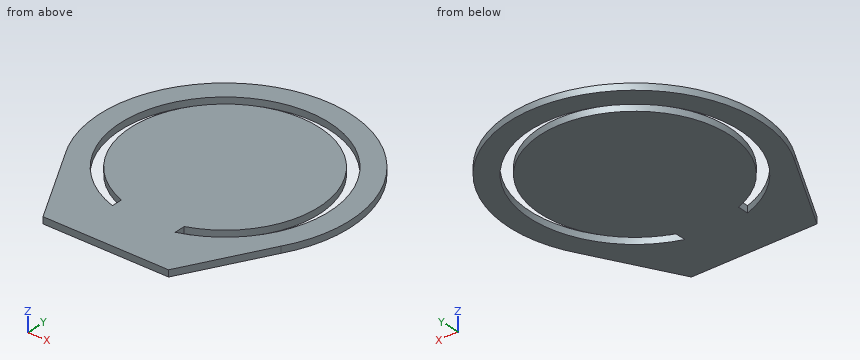
```python
from build123d import *

# Parameters (mm, degrees)
ESBO_O1_R           = 30
ESBO_O1_R_2         = 25
BOSS_EXTRUDE1_DEPTH = 1.57
BOSS_EXTRUDE2_START = -1.57
BOSS_EXTRUDE2_DEPTH = 1.57
BOSS_EXTRUDE3_DEPTH = 1.57
BOSS_EXTRUDE4_START = -1.57
SKETCH4_R           = 22.5
BOSS_EXTRUDE4_DEPTH = 1.57


with BuildPart() as part:
    # Esboço1 → Boss-Extrude1 (new body)
    with BuildSketch(Plane.XY):
        Circle(ESBO_O1_R)
        Circle(ESBO_O1_R_2, mode=Mode.SUBTRACT)
    extrude(amount=BOSS_EXTRUDE1_DEPTH)

    # Sketch1 → Boss-Extrude2 (add)
    with BuildSketch(Plane.XY.offset(1.57).offset(BOSS_EXTRUDE2_START)):
        with BuildLine():
            Line((-25.800536663, -15.307916512), (-15, -35))
            Line((-15, -35), (-15, -25.980762114))
            ThreePointArc((-15, -25.980762114), (-21.086686707, -21.338970071), (-25.800536663, -15.307916512))
        make_face()
        with BuildLine():
            Line((-15, -35), (0, -35))
            Line((0, -35), (0, -30))
            ThreePointArc((0, -30), (-7.764571353, -28.977774789), (-15, -25.980762114))
            Line((-15, -25.980762114), (-15, -35))
        make_face()
        with BuildLine():
            Line((0, -35), (15, -35))
            Line((15, -35), (15, -25.980762114))
            ThreePointArc((15, -25.980762114), (7.764571353, -28.977774789), (0, -30))
            Line((0, -30), (0, -35))
        make_face()
        with BuildLine():
            Line((15, -25.980762114), (15, -35))
            Line((15, -35), (25.800536663, -15.307916512))
            ThreePointArc((25.800536663, -15.307916512), (21.086686707, -21.338970071), (15, -25.980762114))
        make_face()
    extrude(amount=BOSS_EXTRUDE2_DEPTH)

    # Sketch2 → Boss-Extrude3 (add)
    with BuildSketch(Plane.XY):
        with BuildLine():
            ThreePointArc((7.5, -21.213203436), (0, -22.5), (-7.5, -21.213203436))
            Line((-7.5, -21.213203436), (-7.5, -25))
            Line((-7.5, -25), (-2.5, -25))
            Line((-2.5, -25), (2.5, -25))
            Line((2.5, -25), (7.5, -25))
            Line((7.5, -25), (7.5, -21.213203436))
        make_face()
    extrude(amount=BOSS_EXTRUDE3_DEPTH)

    # Sketch4 → Boss-Extrude4 (add)
    with BuildSketch(Plane.XY.offset(1.57).offset(BOSS_EXTRUDE4_START)):
        Circle(SKETCH4_R)
    extrude(amount=BOSS_EXTRUDE4_DEPTH)


solid = part.part
```
Part model, mm, in its own coordinate system. Give positions to 0.01 mm unless a question says otherwise; leave off trailing zeros. Order: outer loops, then holes, each group sorted by start corner. A loop starts at its lowest first (then second) coordinate and runs counter-clockwise, first axis right, second up. Notation, with made-up numbers: M -8.75,19 L 2.25,19 A23 ccw 2.25,54 Z; hole C 70,-35 d8. An arc over 180 degrees is marked long. Use a Markdown table: item, result. Add a question column.
(1) Probe line 1 along X through (y, z) = (0, 0.55); line 2 along X through (y, z) = (4, 1.35); line 3 along Y through (x, z) = (0, 1.05). List the from-to ranges inside material, lowest first. Write a range as [from, to].
(2) Saw through at B-B, the plane y = 0. Give the cut face in (x, z).
(3) Drop flat-ended pins along their axis: P1, Ø0.5, axis at y = -23, z = 1, coming from the +X side; P2, Ø0.5, axis at y = -23, z = 1, coming from the -X side. Give the stop position or say it passes through.
(4) Saw through at A-A, the plane z = 0.35. Give the cut face in (x, y), and give its area (3 significant figures).
(5) Saw through at C-C, the plane x = 0. Give the cut face in (y, z), and give its area (3 significant figures).
(6) Saw through at D-D, the plane y = -11. Give the cut face in (x, z), and give its area (3 significant figures).
Answer key:
| question | item | result |
|---|---|---|
| 1 | line 1 | [-30, -25], [-22.5, 22.5], [25, 30] |
| 1 | line 2 | [-29.73, -24.68], [-22.14, 22.14], [24.68, 29.73] |
| 1 | line 3 | [-35, 22.5], [25, 30] |
| 2 | outline | M -30,0 L -25,0 L -25,1.57 L -30,1.57 Z; M -22.5,0 L 22.5,0 L 22.5,1.57 L -22.5,1.57 Z; M 25,0 L 30,0 L 30,1.57 L 25,1.57 Z |
| 3 | P1 | x = 21.72 |
| 3 | P2 | x = -21.72 |
| 4 | outline | M -25.8,-15.31 L -15,-35 L 15,-35 L 25.8,-15.31 A30 ccw long Z; hole M -7.5,-23.85 L -7.5,-21.21 A22.5 cw long 7.5,-21.21 L 7.5,-23.85 A25 ccw long Z |
| 4 | area | 2,760 mm^2 |
| 5 | outline | M -35,0 L 22.5,0 L 22.5,1.57 L -35,1.57 Z; M 25,0 L 30,0 L 30,1.57 L 25,1.57 Z |
| 5 | area | 98.1 mm^2 |
| 6 | outline | M -27.91,0 L -22.45,0 L -22.45,1.57 L -27.91,1.57 Z; M -19.63,0 L 19.63,0 L 19.63,1.57 L -19.63,1.57 Z; M 22.45,0 L 27.91,0 L 27.91,1.57 L 22.45,1.57 Z |
| 6 | area | 78.8 mm^2 |
